The model under review builds one solid part; all positions refer to its coordinate system, in mm. Face numbers are marked on the shaded views. A direction names the side the tool comes from. Coordinates: 2 decimals unless noted, no trailing zeros. Write each loop counter-clockwise with the first axis right and the second up, starting at its lowest first coordinate (ties: lowest second). Pieces come first, ordered by that corner, then holes. Notation, with made-up numbers: (-36, -20.75) - (-25, -20.75) arc R12 ccw to (-25, -10.75) - close; hole circle Ø10 at (74, 14). An arc over 180 degrees is marked (long way). Put each result on its own line as item: value. Start each with the question number.
Item 1: Consider section A-A on y = 16.5. Give the boundary of the cut face in (x, z), then the cut area to 3 significant figures.
Item 2: Consider section B-B on x = 9.75. Give the boundary of the cut face in (y, z).
Item 3: To check wall thickness, follow L1, parallel to Z at x = 7.5, y = 16.65; L2, parallel to Y at x = 6, z = -14; L3, parallel to Z at x = 7.5, y = 12.5. State the ranges of each line that lie inside material, in increasing order. Write a range as [from, to].
Item 4: Consider section C-C on y = -0.5. Give the boundary of the cut face in (x, z).
Item 5: Consider section D-D on z = -7.5. Give the boundary of the cut face in (x, y).
Item 6: Mouldability with a two-part tool opening along Z and no side actions: class the marked faces 1, 2, 3 and 4 as pulls with the +Z half, pulls with the -Z half, needs draft (parallel to the pull), parting line crosses it, or undercut.
Item 7: For pin 1 (8 mm diameter, centred on x = 3, y = 6.5, fed in from +Z); pin 2 (1 mm diameter, centred on x = 2.5, y = -3, fed in from -Z); pin 3 (4.5 mm diameter, centred on x = 7.5, z = -30.5, fed in from -Y); pin 4 (1.8 mm diameter, centred on x = 7.5, z = -35.22, fed in from +Y), all flat-tipped, find the tip position at first contact; note any pin that passes through.
Item 8: Machinability: for the marked faces 5, 6 and 7, which of the approach directions +Z, -Z, +X, -X, +Y, -Y give a long, thin tool a straight path to every point of the face, cutting with its end or side? Answer none if there is none.
```python
from build123d import *

# Parameters (mm, degrees)
F1_DEPTH = 15
F2_R     = 1.5
F3_DEPTH = 5.001


with BuildPart() as f1:
    # F0 (on Right) → F1 (new body)
    with BuildSketch(Plane.YZ):
        Polygon((-24.130502, -17.715111), (-24.130502, 2.284889), (-29.130502, 2.284889), (-29.130502, -22.715111), (13.869498, -22.715111), (13.869498, -42.715111), (18.869498, -42.715111), (18.869498, -17.715111), align=None)
    extrude(amount=F1_DEPTH)

    # F2 (on face) → F3 (cut, through all)
    with BuildSketch(Plane.XZ.offset(-13.869498)):
        with BuildLine():
            ThreePointArc((15, -35.215111), (12.803301, -40.518412), (7.5, -42.715111))
            Line((7.5, -42.715111), (15, -42.715111))
            Line((15, -42.715111), (15, -35.215111))
        make_face()
        with BuildLine():
            ThreePointArc((7.5, -42.715111), (2.196699, -40.518412), (0, -35.215111))
            Line((0, -35.215111), (0, -42.715111))
            Line((0, -42.715111), (7.5, -42.715111))
        make_face()
        with Locations((7.5, -35.215111)):
            Circle(F2_R)
        with Locations((7.5, -28.215111)):
            Circle(F2_R)
    extrude(amount=-F3_DEPTH, mode=Mode.SUBTRACT)


solid = f1.part
```
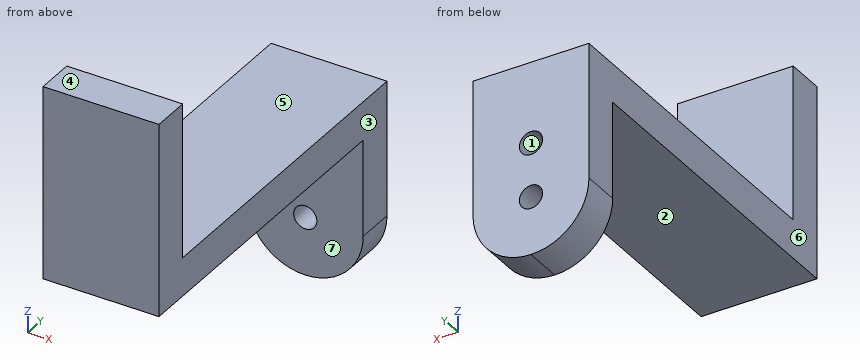
Report:
1. outline: (0, -35.22) arc R7.5 ccw to (15, -35.22) - (15, -17.72) - (0, -17.72) - close; hole circle Ø3 at (7.5, -35.22); hole circle Ø3 at (7.5, -28.22)
1. area: 337 mm²
2. outline: (-29.13, -22.72) - (13.87, -22.72) - (13.87, -42.37) - (18.87, -42.37) - (18.87, -17.72) - (-24.13, -17.72) - (-24.13, 2.28) - (-29.13, 2.28) - close
3. L1: [-42.72, -36.72], [-33.72, -29.72], [-26.72, -17.72]
3. L2: [-29.13, -24.13]
3. L3: [-22.72, -17.72]
4. outline: (0, -22.72) - (15, -22.72) - (15, -17.72) - (0, -17.72) - close
5. outline: (0, -29.13) - (15, -29.13) - (15, -24.13) - (0, -24.13) - close
6. face 1: undercut
6. face 2: pulls with the -Z half
6. face 3: needs draft
6. face 4: pulls with the +Z half
7. pin 1: z = -17.72
7. pin 2: z = -22.72
7. pin 3: y = 13.87
7. pin 4: through
8. face 5: +Z, +X, -X, +Y
8. face 6: +Z, -Z, -X, +Y, -Y
8. face 7: -Z, +X, -X, -Y
